Study the drawing (mm; zero at the part's minimum x, y, z) and answer. Round coordinates to 2 decimals unless told otherwise and drop trailing zeros. Order: outer loops, then holes, each group sorted by start corner. A loop starts at its lowest first (then second) coordinate and runs counter-clockwise, first axis right, second up. Notation, with made-up numbers: M 78.5,-16 L 115.5,-16 A14 cw 115.5,-1 Z; hole C 10.5,10.25 d5. An arc over 180 degrees is marked long. Put each result on its own line as item: value. Start each with the question number.
1. Consider line 1 (X direction, y = 2.75, z = 52); line 2 (X direction, y = 1.85, z = 100); line 3 (X direction, y = 4.6, z = 40). Determine where each line is inside the solid, lowest interval first.
2. The part is cut by section D-D (x = 47). Give the vertices of the cut face in (y, z), then the cut area to 3 significant figures.
3. The part is cut by section B-B (y = 2.75). Give the vertices of the cut face in (x, z), then the cut area to 3 significant figures.
4. The part is cut by section A-A (z = 79). Give the vertices of the cut face in (x, y), then the cut area to 3 significant figures.
5. The part is cut by section C-C (x = 25). Give the vertices of the cut face in (y, z).
6. Each of these flat-tipped pins is pushed along its axis until it touches: pin 1 Ø4.5 at (x, z) = (25, 25) entering from +Y; pin 2 Ø5 at (x, z) = (8.5, 85) entering from -Y; pin 3 Ø2 at (x, y) = (29.5, 1) entering from -Z; pin 4 Ø2.5 at (y, z) = (3.5, 61) entering from +X. Where does it stop, or does it pass through?
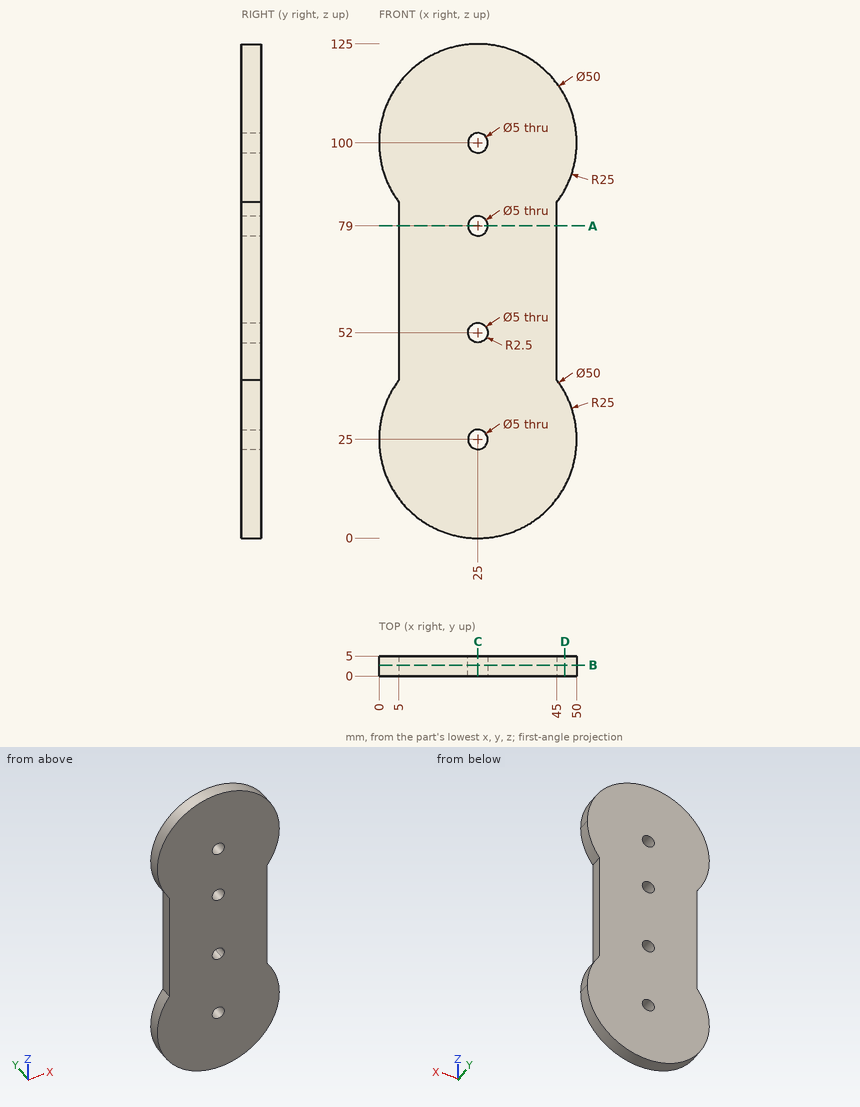
Resolved:
1. line 1: 5 to 22.5, 27.5 to 45
1. line 2: 0 to 22.5, 27.5 to 50
1. line 3: 5 to 45
2. outline: M 0,13.13 L 5,13.13 L 5,36.87 L 0,36.87 Z; M 0,88.13 L 5,88.13 L 5,111.87 L 0,111.87 Z
2. area: 237 mm2
3. outline: M 5,40 A25 ccw long 45,40 L 45,85 A25 ccw long 5,85 Z; hole C 25,25 d5; hole C 25,52 d5; hole C 25,79 d5; hole C 25,100 d5
3. area: 5,090 mm2
4. outline: M 5,0 L 22.5,0 L 22.5,5 L 5,5 Z; M 27.5,0 L 45,0 L 45,5 L 27.5,5 Z
4. area: 175 mm2
5. outline: M 0,0 L 5,0 L 5,22.5 L 0,22.5 Z; M 0,27.5 L 5,27.5 L 5,49.5 L 0,49.5 Z; M 0,54.5 L 5,54.5 L 5,76.5 L 0,76.5 Z; M 0,81.5 L 5,81.5 L 5,97.5 L 0,97.5 Z; M 0,102.5 L 5,102.5 L 5,125 L 0,125 Z
6. pin 1: through
6. pin 2: y = 0
6. pin 3: z = 0.25
6. pin 4: x = 45
